Drawing for the job (mm, zero at the part's lowest x, y, z). Coordinates: 2 decimals unless noted, no trailing zeros. Loops run counter-clockwise (first coordinate to the right, second up) from the corner with the lowest first, then second, coordinate; pieces in that order, holes last. Notation, with made-up numbers: (20, 37) - (39, 37) arc R22 ccw to (39, 66) - close; hole circle Ø8 at (55, 52). An arc over 180 degrees is marked (long way). One line per item, written item: value.
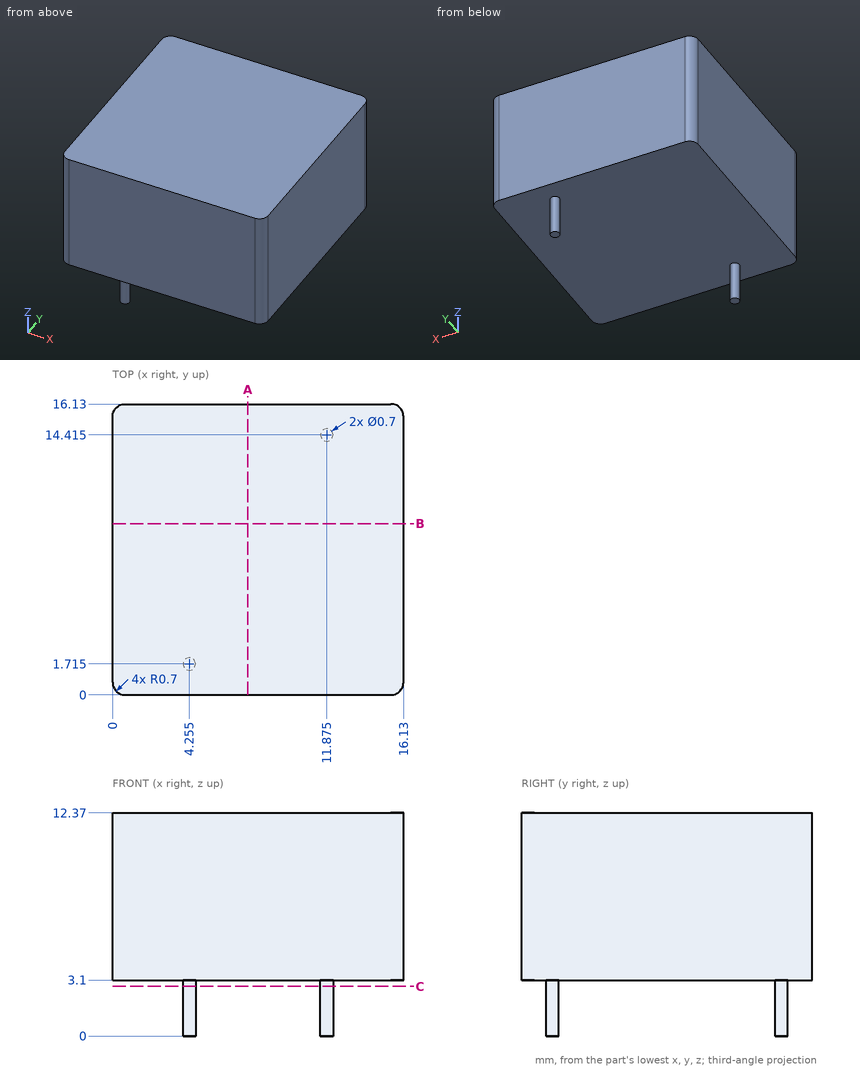
Item 1: Cut at C-C, the plane z = 2.75. Write the cut outline in (x, y) (3 decimals), then the cut area to 3 significant figures.
Check result:
outline: circle Ø0.7 at (4.255, 1.715); circle Ø0.7 at (11.875, 14.415)
area: 0.770 mm^2
Item 2: Cut at A-A, the plane x = 7.5. Write the cut outline in (y, z).
Check result:
outline: (0, 3.1) - (16.13, 3.1) - (16.13, 12.37) - (0, 12.37) - close
Item 3: Drop a flat-ended pin along its axis: P1, Ø5, axis at x = 8.5, y = 9.5, coming from the -Z side. Give the stop position or say it passes through.
Check result:
P1: stops at z = 3.1
Item 4: Probe probe 1 along Z at (x, y) = (10.25, 5.5). List the from-to ranges inside material, lowest first. Write a range as from..to.
Check result:
probe 1: z = 3.1..12.37
